Part model, mm, in its own coordinate system. Give positions to 0.01 mm unless a question says otherwise; leave off trailing zeros. Write each loop counter-clockwise with the first axis right and the second up, starting at its lowest first coordinate (ties: lowest second). Pieces come first, ordered by that corner, then holes. Notation, with made-up numbers: M 29,33 L 66,33 A20 cw 66,57 Z; hole C 64,61.25 d4. An arc over 180 degrees is marked long. Use a Markdown table: item, result.
Autodesk Inventor part; units mm, degrees
ref_plane "YZ Plane" through (0, 0, 0) normal (1, 0, 0) x (0, 1, 0)
ref_plane "XZ Plane" through (0, 0, 0) normal (0, 1, 0) x (-1, 0, 0)
ref_plane "XY Plane" through (0, 0, 0) normal (0, 0, 1) x (1, 0, 0)
sketch "Skizze1" plane through (0, 0, 0) normal (0, 1, 0) x (-1, 0, 0)
  line L0 (2124.7965, -1368.0982) -> (324.7965, -1368.0982)
  line L1 (324.7965, -1368.0982) -> (324.7965, -3168.0982)
  line L2 (324.7965, -3168.0982) -> (2124.7965, -3168.0982)
  line L3 (2124.7965, -3168.0982) -> (2124.7965, -1368.0982)
  line L4 (309.7965, -1353.0982) -> (2139.7965, -1353.0982)
  line L5 (2139.7965, -1353.0982) -> (2139.7965, -3183.0982)
  line L6 (2139.7965, -3183.0982) -> (309.7965, -3183.0982)
  line L7 (309.7965, -3183.0982) -> (309.7965, -1353.0982)
  line L8 (309.7965, -1353.0982) -> (2139.7965, -3183.0982) construction
  line L9 (2139.7965, -1353.0982) -> (309.7965, -3183.0982) construction
  point P0 (0, 0)
  point P1 (1224.7965, -2268.0982)
  dimension "d0" = 1800
  dimension "d1" = 1800
  dimension "d2" = 15
  dimension "d3" = 15
  dimension "d4" = 15
  dimension "d5" = 15
extrude "Extrusion1" add sketch "Skizze1" along normal blind 15
properties part number "Rahmen"
1. Cut at C-C, the plane y = 12.5. Give the cut face in (x, z), then the cut area to 3 significant figures.
Findings below:
| item | result |
|---|---|
| outline | M -2139.8,-3183.1 L -309.8,-3183.1 L -309.8,-1353.1 L -2139.8,-1353.1 Z; hole M -2124.8,-3168.1 L -324.8,-3168.1 L -324.8,-1368.1 L -2124.8,-1368.1 Z |
| area | 109,000 mm2 |
2. Drill centre lines: L1, parallel to X at y = 0.75, z = -2659; L2, parallel to Z at x = -1652, y = 13.5. Where is each one in solid material? Low to high.
Findings below:
| item | result |
|---|---|
| L1 | -2139.8 to -2124.8, -324.8 to -309.8 |
| L2 | -3183.1 to -3168.1, -1368.1 to -1353.1 |
3. Cut at B-B, the plane z = -1804. Give the cut face in (x, y).
Findings below:
| item | result |
|---|---|
| outline | M -2139.8,0 L -2124.8,0 L -2124.8,15 L -2139.8,15 Z; M -324.8,0 L -309.8,0 L -309.8,15 L -324.8,15 Z |
4. Cut at A-A, the plane x = -1168. Give the cut face in (y, z), then the cut area to 3 significant figures.
Findings below:
| item | result |
|---|---|
| outline | M 0,-3183.1 L 15,-3183.1 L 15,-3168.1 L 0,-3168.1 Z; M 0,-1368.1 L 15,-1368.1 L 15,-1353.1 L 0,-1353.1 Z |
| area | 450 mm2 |
